Here's how the part is built. I have some questions about the finished solid (model axes, mm). A direction names the side the tool comes from. Round coordinates to 2 decimals unless told otherwise and drop trailing zeros. Loops run counter-clockwise (first coordinate to the right, second up) from the corner with the lowest first, then second, coordinate; pieces in that order, holes last. Notation, with made-up numbers: M -12.75,88.25 L 23.25,88.25 A21 ccw 23.25,107.25 Z; hole C 39.5,55 d4. An arc over 180 degrees is marked long. Answer as CSV lines item,"result".
```python
from build123d import *

# Parameters (mm, degrees)
SKETCH1_W             = 115.5
SKETCH1_H             = 103.5
CELL_BODY_DEPTH       = 10.625
SKETCH2_W             = 9
SKETCH2_H             = 6
SCREW_TERMINALS_DEPTH = 2
SKETCH3_R             = 2
SCREWS_DEPTH          = 12


with BuildPart() as part:
    # Sketch1 → Cell Body (new, symmetric)
    with BuildSketch(Plane.XY):
        Rectangle(SKETCH1_W, SKETCH1_H)
    extrude(amount=CELL_BODY_DEPTH, both=True)

    # Sketch2 → Screw Terminals (add)
    with BuildSketch(Plane(origin=(0, 51.75, 0), x_dir=(1, 0, 0), z_dir=(0, 1, 0))):
        with Locations((-39.7, 0)):
            Rectangle(SKETCH2_W, SKETCH2_H)
        with Locations((39.7, 0)):
            Rectangle(SKETCH2_W, SKETCH2_H)
    extrude(amount=SCREW_TERMINALS_DEPTH)

    # Sketch3 → Screws (add)
    with BuildSketch(Plane(origin=(0, 53.75, 0), x_dir=(1, 0, 0), z_dir=(0, 1, 0))):
        with Locations(Location((-39.7, 0, 0), (0, 0, 270))):
            Circle(SKETCH3_R)
        with Locations(Location((39.7, 0, 0), (0, 0, 90))):
            Circle(SKETCH3_R)
    extrude(amount=SCREWS_DEPTH)


solid = part.part
```
1. We'd pull the mould along X, two halves only. Please class faces 3 (the flat face through (-42, 53.75, 0)), 4 (the cylindrical face through (37.717, 59.666, 0.26)), 5 (the flat face through (57.75, -1, 0)), 6 (the flat face through (-1, -51.75, 0)): pulls with the +X half, pulls with the -X half, needs draft (parallel to the pull), parting line crosses it, or undercut.
Evaluation:
face 3,"undercut"
face 4,"undercut"
face 5,"pulls with the +X half"
face 6,"needs draft"
2. I want a section at A-A, the plane x = -39.7. Please give me the cut outline in (y, z) (3 decimals), and give its area (3 significant figures).
Evaluation:
outline,"M -51.75,-10.625 L 51.75,-10.625 L 51.75,-3 L 53.75,-3 L 53.75,-2 L 65.75,-2 L 65.75,2 L 53.75,2 L 53.75,3 L 51.75,3 L 51.75,10.625 L -51.75,10.625 Z"
area,"2,260 mm²"
3. I want a section at C-C, the plane x = 15.5. Please give me the cut outline in (y, z) (3 decimals).
Evaluation:
outline,"M -51.75,-10.625 L 51.75,-10.625 L 51.75,10.625 L -51.75,10.625 Z"
4. Which directions (+Z, -Z, +X, -X, +Y, -Y) give clear straight access to the entire face, cutting with the end or side of a thin tool? Please do faces 1 (the flat face through (-1, 1, -10.625)), 2 (the cylindrical face through (-37.717, 59.666, -0.26)).
Evaluation:
face 1,"-Z, +X, -X, +Y, -Y"
face 2,"+Y"
5. For P1, Ø3, axis at x = -36.5, z = 4, coming from the +Y side; P2, Ø6.5, axis at x = -19, z = 4.5, coming from the +Y side; P3, Ø1, axis at y = 53, z = 0, coming from the +X side, each with a flat end and sliding along its axis, tell me the tip position at first contact or that it passes through.
Evaluation:
P1,"stops at y = 53.75"
P2,"stops at y = 51.75"
P3,"stops at x = 44.2"
6. I want a section at B-B, the plane z = 0. Please give me the cut outline in (x, y).
Evaluation:
outline,"M -57.75,-51.75 L 57.75,-51.75 L 57.75,51.75 L 44.2,51.75 L 44.2,53.75 L 41.7,53.75 L 41.7,65.75 L 37.7,65.75 L 37.7,53.75 L 35.2,53.75 L 35.2,51.75 L -35.2,51.75 L -35.2,53.75 L -37.7,53.75 L -37.7,65.75 L -41.7,65.75 L -41.7,53.75 L -44.2,53.75 L -44.2,51.75 L -57.75,51.75 Z"
7. I want a section at D-D, the plane z = 7.5. Please give me the cut outline in (x, y).
Evaluation:
outline,"M -57.75,-51.75 L 57.75,-51.75 L 57.75,51.75 L -57.75,51.75 Z"
8. If I drill on line 1 (Y direction, x = 43, z = -0.5); line 2 (Y direction, x = -5, z = -0.5), over which ranges is the centre line in solid material (lowest first)? Write a range as [from, to].
Evaluation:
line 1,"y = [-51.75, 53.75]"
line 2,"y = [-51.75, 51.75]"
